Read the model definition and answer for the solid it produces. Units are mm, in the model's axes. A direction names the side the tool comes from. Round coordinates to 2 decimals unless told otherwise and drop trailing zeros. Write each loop counter-clockwise with the first axis right and the second up, starting at its lowest first coordinate (ties: lowest second). Pieces come first, ordered by that corner, then holes.
from build123d import *

# Parameters (mm, degrees)
F1_DEPTH = 12.5


with BuildPart() as f1:
    # F0 (on Top) → F1 (new body)
    with BuildSketch(Plane.XY):
        with BuildLine():
            Line((0, 8), (0, 0))
            Line((0, 0), (20, 0))
            Line((20, 0), (21, -5))
            Line((21, -5), (21, -8))
            ThreePointArc((21, -8), (22.484724, -10.28456), (25.175371, -9.855568))
            Line((25.175371, -9.855568), (29.114077, -6.299355))
            ThreePointArc((29.114077, -6.299355), (29.166714, -6.079108), (28.980047, -5.95091))
            Line((28.980047, -5.95091), (27, -5.95091))
            ThreePointArc((27, -5.95091), (26.292893, -5.658016), (26, -4.95091))
            Line((26, -4.95091), (26, 1.486624))
            ThreePointArc((26, 1.486624), (24.092276, 6.092276), (19.486624, 8))
            Line((19.486624, 8), (0, 8))
        make_face()
    extrude(amount=F1_DEPTH)


solid = f1.part
Q1. Which of the six approach directions +Z, -Z, +X, -X, +Y, -Y give full straight-line access (tool end or side, diameter ignored) to faces 1 (the flat face through (10, 8, 6)), 2 (the flat face through (26, -2, 6)), 3 (the flat face through (21, -6, 6))?
Verdict:
face 1: +Z, -Z, +X, -X, +Y
face 2: +Z, -Z, +X, +Y
face 3: +Z, -Z, -X, -Y
Q2. Section A-A (z = 1) is taken. Determine the outline of the cut face in (x, y), then the cut area to 3 significant figures.
Verdict:
outline: (0, 0) - (20, 0) - (21, -5) - (21, -8) arc R2.5 ccw to (25.18, -9.86) - (29.11, -6.3) arc R0.2 ccw to (28.98, -5.95) - (27, -5.95) arc R1 cw to (26, -4.95) - (26, 1.49) arc R6.51 ccw to (19.49, 8) - (0, 8) - close
area: 257 mm2
Q3. Section C-C (x = 9.75) is taken. Determine the outline of the cut face in (y, z), then the cut area to 3 significant figures.
Verdict:
outline: (0, 0) - (8, 0) - (8, 12.5) - (0, 12.5) - close
area: 100 mm2
Q4. Flat-ended cylindrical pins translate along their axes: pin 1 Ø7 at (y, z) = (-0.5, 5.5) entering from +X; pin 2 Ø2 at (x, z) = (24, 3.5) entering from +Y; pin 3 Ø5 at (y, z) = (-1.5, 11) entering from -X; pin 4 Ø1 at (x, z) = (28, 4.5) entering from +Y. Find the tip coordinate at first contact, or state that the pin passes through.
Verdict:
pin 1: stops at x = 26
pin 2: stops at y = 6.97
pin 3: stops at x = 0
pin 4: stops at y = -5.95
Q5. Straight lines are drawn through the part: probe 1 along Y at (x, z) = (10.25, 4.25); probe 2 along X at (y, z) = (-2, 5.5); probe 3 along X at (y, z) = (3.25, 9.5). For each, find the intervals that lie inside material, in ascending order.
Verdict:
probe 1: y = 0 to 8
probe 2: x = 20.4 to 26
probe 3: x = 0 to 25.76
Q6. Section B-B (y = -2.5) is taken. Determine the outline of the cut face in (x, z).
Verdict:
outline: (20.5, 0) - (26, 0) - (26, 12.5) - (20.5, 12.5) - close
